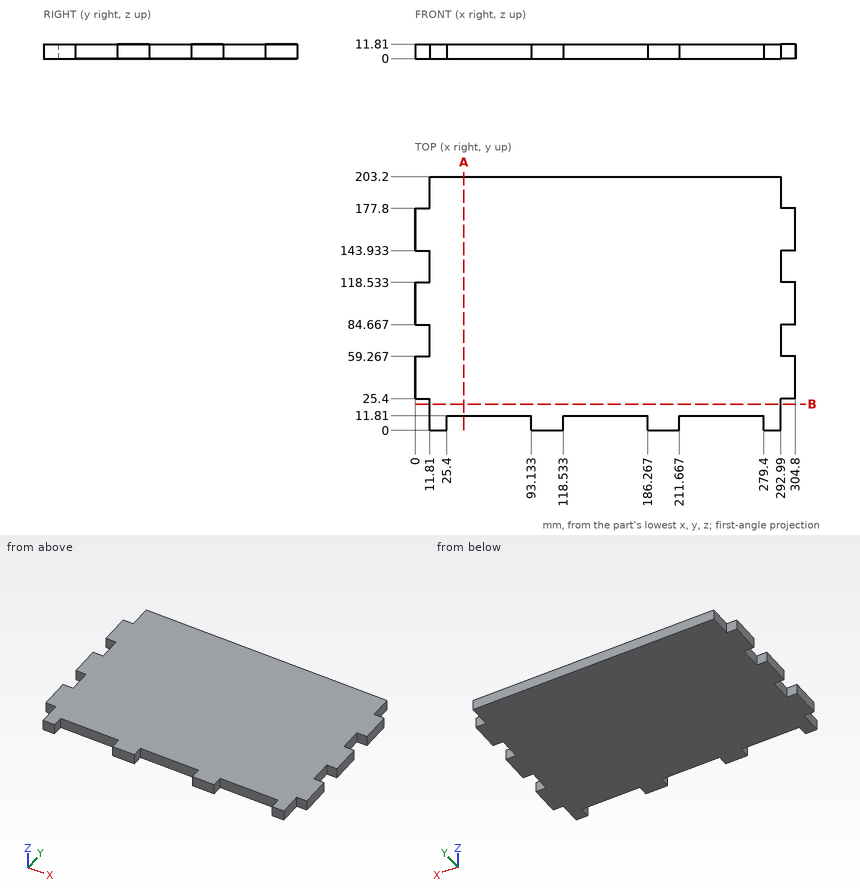
Design review of the part shown in the three views and the two pictorial views. Dimensions are in mm from the part's minimum x, y and z. Coordinates: 2 decimals unless noted, no trailing zeros. Order: outer loops, then holes, each group sorted by start corner. A loop starts at its lowest first (then second) coordinate and runs counter-clockwise, first axis right, second up. Notation, with made-up numbers: (-39, -25.5) -> (10, -25.5) arc R17 ccw to (10, -20.5) -> close; hole circle Ø4 at (64.25, 2). An arc over 180 degrees is marked (long way). Use one line per item in the form item = value. Start each with the question number.
(1) For probe 1 along X at (y, z) = (75.5, 1.5); probe 2 along Y at (x, z) = (79.5, 7), list the stretches that pass through material, from the lowest coordinate up.
(2) Add section A-A on x = 39. State the section outline as (y, z) points.
(3) Insertion check: pin 1 (6 mm diameter, centred on y = 3.5, z = 6.5, fed in from +X); pin 2 (3.5 mm diameter, centred on x = 301.5, z = 8, fed in from +Y); pin 3 (6 mm diameter, centred on x = 5, z = 6.5, fed in from -Y). Each pin has a flat end and moves straight along its axis. Give the tip position at first contact, or say it passes through.
(4) Add section B-B on y = 21. State the section outline as (x, z) points, plus the area to 3 significant figures.
Answer block:
q1.probe_1 = 11.81 to 292.99
q1.probe_2 = 11.81 to 203.2
q2.outline = (11.81, 0) -> (203.2, 0) -> (203.2, 11.81) -> (11.81, 11.81) -> close
q3.pin_1 = 292.99
q3.pin_2 = 177.8
q3.pin_3 = 25.4
q4.outline = (11.81, 0) -> (292.99, 0) -> (292.99, 11.81) -> (11.81, 11.81) -> close
q4.area = 3,320 mm²
